Autodesk Inventor part; units mm, degrees
ref_plane "Work Plane1" through (0.75, 0, 0) normal (0, 0, -1) x (1, 0, 0)
ref_plane "YZ Plane" through (0, 0, 0) normal (1, 0, 0) x (0, 1, 0)
ref_plane "XZ Plane" through (0, 0, 0) normal (0, 1, 0) x (-1, 0, 0)
sketch "草图1" plane through (0, 0, 0) normal (0, 0, 1) x (1, 0, 0)
  line L0 (-0.580263, 0) -> (3.481577, 0)
  line L1 (0, 3.8) -> (0, 13.95)
  line L2 (0, 42.332542) -> (3.575394, 50)
  line L3 (3.575394, 50) -> (4.934856, 49.366073)
  line L4 (4.934856, 49.366073) -> (1.5, 42)
  line L5 (1.5, 42) -> (1.5, 32.5)
  line L6 (1.5, 32.5) -> (0, 32.5)
  dimension "d1" = 1.5
  dimension "d2" = 65
  dimension "d3" = 84
  dimension "d4" = 100
  dimension "d5" = 25
  dimension "d6" = 1.5
sketch "草图1 outline for 轴承体" plane through (0, 0, 0) normal (0, 0, 1) x (1, 0, 0)
  line L0 (3.575394, 50) -> (0, 42.332542)
  line L1 (4.934856, 49.366073) -> (3.575394, 50)
  line L2 (1.5, 42) -> (4.934856, 49.366073)
  line L3 (1.5, 32.5) -> (1.5, 42)
  line L4 (0, 32.5) -> (1.5, 32.5)
  line L5 (0, 42.332542) -> (0, 32.5)
revolve "轴承体" add sketch "草图1 outline for 轴承体" angle 360 about axis through (-10, 0, 0) along (1, 0, 0)
sketch "草图2" plane through (0, 0, 0) normal (-1, 0, 0) x (0, 0, 1)
  line L0 (0, -70) -> (0, 70)
  line L1 (3.85, 32.271156) -> (3.85, 28.5)
  line L2 (3.85, 28.5) -> (0, 28.5)
  line L3 (-3.85, 32.271156) -> (-3.85, 28.5)
  line L4 (-3.85, 28.5) -> (0, 28.5)
  line L5 (-70, 0) -> (70, 0)
  circle A0 centre (0, 0) radius 32.5
  circle A1 centre (0, 0) radius 50
  circle A2 centre (0, 0) radius 42
  line L6 (-3.85, 30) -> (3.85, 30)
  circle A3 centre (0, 0) radius 42.332542
  line L7 (3.85, 41.823169) -> (3.85, 49.851555)
  line L8 (0, 70) -> (0, -70)
  line L9 (0, 0) -> (25, 43.30127) construction
  line L10 (17.577387, 38.144927) -> (21.59158, 45.097713)
  line L11 (24.245783, 34.294927) -> (28.259975, 41.247713)
  line L12 (-3.85, 41.823169) -> (-3.85, 49.851555)
  line L13 (0, 0) -> (43.30127, 25) construction
  line L14 (34.294927, 24.245783) -> (41.247713, 28.259975)
  line L15 (38.144927, 17.577387) -> (45.097713, 21.59158)
  line L16 (0, 0) -> (-48.296291, -12.940952) construction
  line L17 (-41.394533, -7.105818) -> (-49.149357, -9.183717)
  line L18 (-39.401626, -14.543447) -> (-47.156451, -16.621346)
  line L19 (0, 0) -> (-35.355339, -35.355339) construction
  line L20 (0, 0) -> (-12.940952, -48.296291) construction
  line L21 (-32.295808, -26.851086) -> (-37.972733, -32.528011)
  line L22 (-26.851086, -32.295808) -> (-32.528011, -37.972733)
  line L23 (-14.543447, -39.401626) -> (-16.621346, -47.156451)
  line L24 (-7.105818, -41.394533) -> (-9.183717, -49.149357)
  dimension "d9" = 7.7
  dimension "d21" = 1.5
  dimension "d25" = 61
  dimension "d32" = 7.7
  dimension "d34" = 7.7
  dimension "d36" = 30
  dimension "d38" = 3.85
  dimension "d39" = 30
  dimension "d40" = 15
  dimension "d41" = 7.7
  dimension "d42" = 30
  dimension "d43" = 30
  dimension "d45" = 7.7
  dimension "d47" = 7.7
sketch "草图2 outline for 切口" plane through (0, 0, 0) normal (-1, 0, 0) x (0, 0, 1)
  arc A0 (-14.543447, -39.401626) -> (-26.851086, -32.295808) centre (0, 0) cw
  line L0 (-16.621346, -47.156451) -> (-14.543447, -39.401626)
  arc A1 (-32.528011, -37.972733) -> (-16.621346, -47.156451) centre (0, 0) ccw
  line L1 (-26.851086, -32.295808) -> (-32.528011, -37.972733)
  arc A2 (-32.295808, -26.851086) -> (-39.401626, -14.543447) centre (0, 0) cw
  line L2 (-37.972733, -32.528011) -> (-32.295808, -26.851086)
  arc A3 (-47.156451, -16.621346) -> (-37.972733, -32.528011) centre (0, 0) ccw
  line L3 (-39.401626, -14.543447) -> (-47.156451, -16.621346)
  line L4 (3.85, 49.851555) -> (3.85, 41.823169)
  arc A4 (21.59158, 45.097713) -> (3.85, 49.851555) centre (0, 0) ccw
  line L5 (17.577387, 38.144927) -> (21.59158, 45.097713)
  arc A5 (3.85, 41.823169) -> (17.577387, 38.144927) centre (0, 0) cw
  line L6 (28.259975, 41.247713) -> (24.245783, 34.294927)
  arc A6 (41.247713, 28.259975) -> (28.259975, 41.247713) centre (0, 0) ccw
  line L7 (34.294927, 24.245783) -> (41.247713, 28.259975)
  arc A7 (24.245783, 34.294927) -> (34.294927, 24.245783) centre (0, 0) cw
  arc A8 (-41.394533, -7.105818) -> (-3.85, 41.823169) centre (0, 0) cw
  line L8 (-49.149357, -9.183717) -> (-41.394533, -7.105818)
  arc A9 (-3.85, 49.851555) -> (-49.149357, -9.183717) centre (0, 0) ccw
  line L9 (-3.85, 41.823169) -> (-3.85, 49.851555)
  line L10 (45.097713, 21.59158) -> (38.144927, 17.577387)
  arc A10 (-9.183717, -49.149357) -> (45.097713, 21.59158) centre (0, 0) ccw
  line L11 (-7.105818, -41.394533) -> (-9.183717, -49.149357)
  arc A11 (38.144927, 17.577387) -> (-7.105818, -41.394533) centre (0, 0) cw
extrude "切口" cut sketch "草图2 outline for 切口" against normal through all
extrude "榫1" add sketch "草图2" against normal blind 1.5 contours L4 L3 L6 L0 | L0 L6 L1 L2 | A0 L0 L6 L3 | L1 L6 L0 A0
extrude "榫2" add sketch "草图2" against normal blind 6 contours L4 L3 L6 L0 | L0 L6 L1 L2
ref_plane "Work Plane1" through (0.75, 0, 0) normal (0, 0, -1) x (1, 0, 0)
equation "\"d1\" = SD"
equation "\"d2\" = SD1"
equation "\"d3\" = LADI"
equation "\"d4\" = SD2"
equation "\"d5\" = FAWI"
equation "\"d6\" = SD"
equation "\"d9\" = TW0"
equation "\"d21\" = SD"
equation "\"d25\" = SD3"
equation "\"d32\" = TW0"
equation "\"d34\" = TW0"
equation "\"d36\" = SEWI"
equation "\"d39\" = SEWI"
equation "\"d40\" = ANG1"
equation "\"d41\" = TW0"
equation "\"d42\" = SEWI"
equation "\"d43\" = SEWI"
equation "\"d45\" = TW0"
equation "\"d47\" = TW0"
equation "\"d17\" = SD"
equation "\"d13\" = SD"
equation "\"d23\" = TL1"
equation "\"FAWI\" = 25deg"
equation "\"SD1\" = 65"
equation "\"SD2\" = 100"
equation "\"SD\" = 1.5"
equation "\"TW0\" = 7.7"
equation "\"LADI\" = 84"
equation "\"d8\" = SD1"
equation "\"TL1\" = 6"
equation "\"SD3\" = 61"
equation "\"SEWI\" = 30deg"
equation "\"ANG1\" = 15deg"
equation "\"RR\" = 0.1"
equation "\"NND\" = 64"
equation "\"PB\" = TW0"
equation "\"PNT\" = TL1"
properties part number "垫圈 GB 858 64" material "钢，软"
Can you work these out from the model? Positions are in its coordinate system, mm. A direction names the side the tool comes from. Coordinates: 2 decimals unless noted, no trailing zeros. Loops run counter-clockwise (first coordinate to the right, second up) from the corner with the lowest first, then second, coordinate; pieces in that order, holes last. Notation, with made-up numbers: (57, 63.5) - (88, 63.5) arc R34 ccw to (88, 93.5) - close; hole circle Ø6 at (43, 49). An arc over 180 degrees is marked (long way). Put each result on its own line as item: value. Start each with the question number.
Item 1: Suppose I cut it at D-D (z = 30). Please give me the cut outline in (x, y), and give its area (3 significant figures).
Item 2: Suppose I cut it at A-A (z = 0). Please give me the cut outline in (x, y), and give its area (3 significant figures).
Item 3: Suppose I cut it at C-C (x = 2.5). Please give me the cut outline in (y, z).
Item 4: Suppose I cut it at B-B (y = 0). Please give me the cut outline in (x, z).
Item 5: For pin 1 (1.3 mm diameter, centred on x = 4, z = 1.5, fed in from +Y); pin 2 (3 mm diameter, centred on x = 2, z = 0.5, fed in from -Y); pin 3 (3 mm diameter, centred on x = 1, y = -10.5, fed in from -Z), each with a flat end and sliding along its axis, tell me the tip position at first contact or that it passes through.
Item 6: If we mould it in two halves opening along Z, with no side actions, what happens to faces 6 (the face through (4.2, -35.1, -35.2)), 7 (the face through (2.273, 26.095, 37.498)), 8 (the face through (2.456, 19.594, 41.638))? For each: +Z half, -Z half, draft (parallel to the pull), parting line (faces both ways), or undercut.
Item 7: If I drill on line 1 along Z through (x, y) = (0.6, 0); line 2 along X through (y, z) = (-26, -31); line 3 along Z through (x, y) = (1, 16), over which ranges is the centre line in solid material (lowest first)?
Item 8: Which directions (+Z, -Z, +X, -X, +Y, -Y) give clear straight access to the entire face, cutting with the end or side of a thin tool? Please do faces 1 (the face through (2.3, 41.3, 19.4)), 2 (the face through (2.456, -29.703, -35.148)), 3 (the face through (0, 18.3, -27.4)), 4 (the face through (2.27, -15.5, -42.97)), 5 (the face through (2, 46, -3.85)).
Here are the results:
1. outline: (0, -29.39) - (1.5, -29.39) - (1.5, -12.5) - (0, -12.5) - close; (0, 12.5) - (1.5, 12.5) - (1.5, 29.39) - (0, 29.39) - close
1. area: 50.7 mm²
2. outline: (0, -42) - (1.5, -42) - (1.5, -32.5) - (0, -32.5) - close; (0, 28.5) - (6, 28.5) - (6, 30) - (1.5, 30) - (1.5, 42) - (4.93, 49.37) - (3.58, 50) - (0, 42.33) - close
2. area: 53.9 mm²
3. outline: (-46.91, -8.58) arc R47.69 ccw to (-44.92, -16.02) - (-41.48, -15.1) arc R44.14 cw to (-43.47, -7.66) - close; (-36.34, -30.89) arc R47.69 ccw to (-30.89, -36.34) - (-28.37, -33.82) arc R44.14 cw to (-33.82, -28.37) - close; (-16.02, -44.92) arc R47.69 ccw to (-8.58, -46.91) - (-7.66, -43.47) arc R44.14 cw to (-15.1, -41.48) - close; (18.65, 40.01) arc R44.14 cw to (25.32, 36.16) - (27.1, 39.24) arc R47.69 ccw to (20.43, 43.09) - close; (28.5, -3.85) - (30, -3.85) - (30, 3.85) - (28.5, 3.85) - close; (36.16, 25.32) arc R44.14 cw to (40.01, 18.65) - (43.09, 20.43) arc R47.69 ccw to (39.24, 27.1) - close; (43.98, -3.85) - (47.54, -3.85) arc R47.69 ccw to (47.54, 3.85) - (43.98, 3.85) arc R44.14 cw to start
4. outline: (0, -42) - (1.5, -42) - (1.5, -32.5) - (0, -32.5) - close; (0, 32.5) - (1.5, 32.5) - (1.5, 42) - (0, 42) - close
5. pin 1: y = 49.99
5. pin 2: y = -42
5. pin 3: z = -46.54
6. face 6: -Z half
6. face 7: undercut
6. face 8: +Z half
7. line 1: -42 to -32.5, 32.5 to 42
7. line 2: 0 to 1.5
7. line 3: -38.83 to -28.29, 28.29 to 38.83
8. face 1: +X, -X, +Y
8. face 2: -Z, +X, -X
8. face 3: +Z, -Z, -X, +Y, -Y
8. face 4: +X, -X, -Y
8. face 5: -Z, +X, -X, +Y
